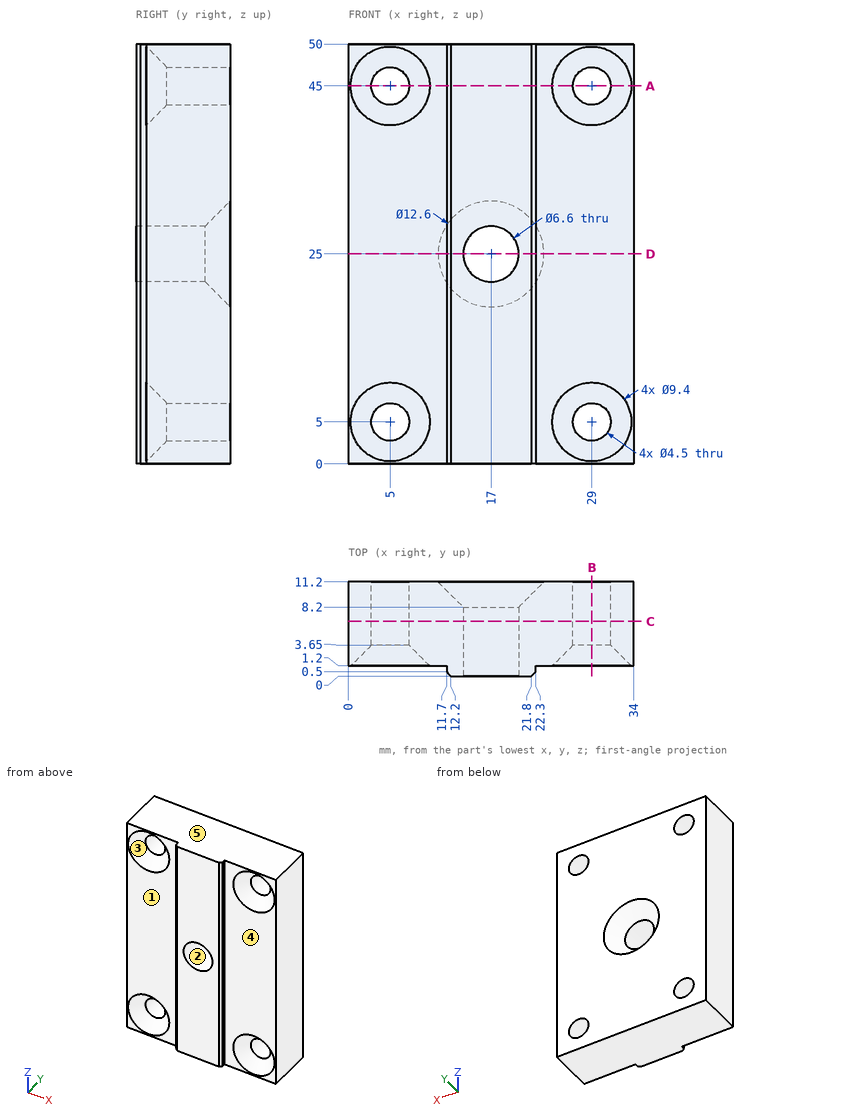
The drawing under review shows one solid part. Ordinate dimensions are in mm from its lowest x, y, z. A direction names the side the tool comes from. Give positions to 0.01 mm unless a question says otherwise; leave off trailing zeros. Loops run counter-clockwise (first coordinate to the right, second up) from the corner with the lowest first, then second, coordinate; pieces in that order, holes last. Notation, with made-up numbers: M -14,62 L -7,62 A34 cw -7,99 Z; hole C 78,-2.5 d10. An arc over 180 degrees is marked long. One line per question, with ' | ' between items. Start each with the question number.
1. The part is to be moulded in two halves that separate along Z. For the marked faces 3, 4 and 5, say which applies: released by +Z, released by -Z, zero draft, split by the parting line, or undercut.
2. Add section D-D (z = 25). Write out the cut boundary in (x, y).
3. Add section B-B (x = 29). Write out the cut boundary in (y, z).
4. Add section A-A (z = 45). Write out the cut boundary in (x, y), plus the area to 3 significant figures.
5. For the marked faces 1 and 2, list the 3-axis set-ups (+Z, -Z, +X, -X, +Y, -Y) from which the entire face can be reached by the end or side of a thin tool; tool diameter is ignored.
6. Insertion check: P1, Ø12, axis at x = 28.5, z = 36.5, coming from the -Y side; P2, Ø4, axis at x = 30, z = 6, coming from the -Y side; P3, Ø8, axis at x = 26, z = 32, coming from the -Y side. Each pin has a flat end and moves straight along its axis. Give the tip position at first contact, or say it passes through.
7. Add section C-C (y = 6.5). Write out the cut boundary in (x, z), plus the area to 3 significant figures.
8. To check wall thickness, follow L1, parallel to Z at x = 5, y = 7; L2, parallel to X at y = 4.5, z = 45; L3, parallel to X at y = 6.25, z = 6.5. State the ranges of each line that lie inside material, in increasing order.
Worked out:
1) face 3: undercut | face 4: zero draft | face 5: released by +Z
2) outline: M 0,1.2 L 11.7,1.2 L 11.7,0.5 L 12.2,0 L 13.7,0 L 13.7,8.2 L 10.7,11.2 L 0,11.2 Z; M 20.3,0 L 21.8,0 L 22.3,0.5 L 22.3,1.2 L 34,1.2 L 34,11.2 L 23.3,11.2 L 20.3,8.2 Z
3) outline: M 1.2,0 L 11.2,0 L 11.2,2.75 L 3.65,2.75 L 1.2,0.3 Z; M 1.2,9.7 L 3.65,7.25 L 11.2,7.25 L 11.2,42.75 L 3.65,42.75 L 1.2,40.3 Z; M 1.2,49.7 L 3.65,47.25 L 11.2,47.25 L 11.2,50 L 1.2,50 Z
4) outline: M 0,1.2 L 0.3,1.2 L 2.75,3.65 L 2.75,11.2 L 0,11.2 Z; M 7.25,3.65 L 9.7,1.2 L 11.7,1.2 L 11.7,0.5 L 12.2,0 L 21.8,0 L 22.3,0.5 L 22.3,1.2 L 24.3,1.2 L 26.75,3.65 L 26.75,11.2 L 7.25,11.2 Z; M 31.25,3.65 L 33.7,1.2 L 34,1.2 L 34,11.2 L 31.25,11.2 Z | area: 250 mm²
5) face 1: +Z, -Z, -X, -Y | face 2: +Y, -Y
6) P1: stops at y = 1.2 | P2: stops at y = 2.49 | P3: stops at y = 0.2
7) outline: M 0,0 L 34,0 L 34,50 L 0,50 Z; hole C 5,5 d4.5; hole C 5,45 d4.5; hole C 17,25 d6.6; hole C 29,5 d4.5; hole C 29,45 d4.5 | area: 1,600 mm²
8) L1: z = 0 to 2.75, 7.25 to 42.75, 47.25 to 50 | L2: x = 0 to 2.75, 7.25 to 26.75, 31.25 to 34 | L3: x = 0 to 3.32, 6.68 to 27.32, 30.68 to 34
